Autodesk Fusion 360 part; units mm, degrees
sketch "Skizze1" plane through (0, 0, 0) normal (0, 0, 1) x (1, 0, 0)
  line L0 (0, 0) -> (57, 0)
  line L1 (57, 0) -> (57, 87)
  line L2 (57, 87) -> (0, 87)
  line L3 (0, 87) -> (0, 0)
  dimension "d1" = 57
  dimension "d2" = 87
extrude "Extrusion1" add sketch "Skizze1" along normal blind 1.75
fillet "Abrundung1" radius 2 4 edges at (0, 0, 0.875) (57, 0, 0.875) (57, 87, 0.875) (0, 87, 0.875)
sketch "Skizze2" plane through (0, 0, 1.75) normal (0, 0, 1) x (-1, 0, 0)
  arc A0 (-2, -87) -> (0, -85) centre (-2, -85) ccw
  line L0 (0, -85) -> (0, -2)
  arc A1 (0, -2) -> (-2, 0) centre (-2, -2) ccw
  line L1 (-2, 0) -> (-55, 0)
  arc A2 (-55, 0) -> (-57, -2) centre (-55, -2) ccw
  line L2 (-57, -2) -> (-57, -85)
  arc A3 (-57, -85) -> (-55, -87) centre (-55, -85) ccw
  line L3 (-55, -87) -> (-2, -87)
  line L4 (-5.5896, -49.2464) -> (-5.5896, -40.6115)
  line L5 (-5.5896, -40.6115) -> (-12.2493, -39.4747)
  spline S0 degree 3 poles (-12.2493, -39.4747) (-12.5241, -38.6458) (-12.8509, -37.8501) (-13.2393, -37.0827) knots 0 0 0 0 1 1 1 1
  line L6 (-13.2393, -37.0827) -> (-9.3316, -31.5693)
  line L7 (-9.3316, -31.5693) -> (-15.4418, -25.459)
  line L8 (-15.4418, -25.459) -> (-20.9932, -29.3904)
  spline S1 degree 3 poles (-20.9932, -29.3904) (-21.7416, -29.0162) (-22.5231, -28.7083) (-23.3331, -28.4478) knots 0 0 0 0 1 1 1 1
  line L9 (-23.3331, -28.4478) -> (-24.4794, -21.7171)
  line L10 (-24.4794, -21.7171) -> (-33.1143, -21.7171)
  line L11 (-33.1143, -21.7171) -> (-34.2747, -28.5189)
  spline S2 degree 3 poles (-34.2747, -28.5189) (-35.0515, -28.7794) (-35.7952, -29.092) (-36.5152, -29.4567) knots 0 0 0 0 1 1 1 1
  line L12 (-36.5152, -29.4567) -> (-42.1565, -25.459)
  line L13 (-42.1565, -25.459) -> (-48.2668, -31.5693)
  line L14 (-48.2668, -31.5693) -> (-44.2454, -37.2438)
  spline S3 degree 3 poles (-44.2454, -37.2438) (-44.5959, -37.9495) (-44.8801, -38.679) (-45.1359, -39.4321) knots 0 0 0 0 1 1 1 1
  line L15 (-45.1359, -39.4321) -> (-52.0087, -40.6068)
  line L16 (-52.0087, -40.6068) -> (-52.0087, -49.2464)
  line L17 (-52.0087, -49.2464) -> (-45.1311, -50.4211)
  spline S4 degree 3 poles (-45.1311, -50.4211) (-44.8801, -51.179) (-44.5911, -51.8989) (-44.2406, -52.6047) knots 0 0 0 0 1 1 1 1
  line L18 (-44.2406, -52.6047) -> (-48.262, -58.2839)
  line L19 (-48.262, -58.2839) -> (-42.1565, -64.3895)
  line L20 (-42.1565, -64.3895) -> (-36.5152, -60.3965)
  spline S5 degree 3 poles (-36.5152, -60.3965) (-35.7952, -60.7612) (-35.0515, -61.0691) (-34.2795, -61.3343) knots 0 0 0 0 1 1 1 1
  line L21 (-34.2795, -61.3343) -> (-33.1143, -68.1362)
  line L22 (-33.1143, -68.1362) -> (-24.4746, -68.1362)
  line L23 (-24.4746, -68.1362) -> (-23.3236, -61.4054)
  spline S6 degree 3 poles (-23.3236, -61.4054) (-22.5137, -61.1401) (-21.7368, -60.837) (-20.9885, -60.4628) knots 0 0 0 0 1 1 1 1
  line L24 (-20.9885, -60.4628) -> (-15.4418, -64.3942)
  line L25 (-15.4418, -64.3942) -> (-9.3316, -58.2887)
  line L26 (-9.3316, -58.2887) -> (-13.2346, -52.7752)
  spline S7 degree 3 poles (-13.2346, -52.7752) (-12.8414, -52.0079) (-12.5193, -51.2121) (-12.2446, -50.3832) knots 0 0 0 0 1 1 1 1
  line L27 (-12.2446, -50.3832) -> (-5.5896, -49.2464)
  spline S8 degree 3 poles (-28.695, -53.2157) (-33.2706, -53.2157) (-36.9841, -49.5069) (-36.9841, -44.9266) knots 0 0 0 0 1 1 1 1
  spline S9 degree 3 poles (-36.9841, -44.9266) (-36.9841, -40.351) (-33.2706, -36.6375) (-28.695, -36.6375) knots 0 0 0 0 1 1 1 1
  spline S10 degree 3 poles (-28.695, -36.6375) (-24.1146, -36.6375) (-20.4058, -40.351) (-20.4058, -44.9266) knots 0 0 0 0 1 1 1 1
  spline S11 degree 3 poles (-20.4058, -44.9266) (-20.4058, -49.5069) (-24.1194, -53.2157) (-28.695, -53.2157) knots 0 0 0 0 1 1 1 1
extrude "Extrusion2" cut sketch "Skizze2" against normal blind 0.4 contours L4 L5 S0 L6 L7 L8 S1 L9 L10 L11 S2 L12 L13 L14 S3 L15 L16 L17 S4 L18 L19 L20 S5 L21 L22 L23 S6 L24 L25 L26 S7 L27
extrude "Extrusion3" cut 1 faces at (19, 57.3333, 0) along direction (0, 0, 1) blind 0.2
extrude "Extrusion4" cut 1 faces at (19, 57.3333, 0.2) along direction (0, 0, 1) blind 0.05
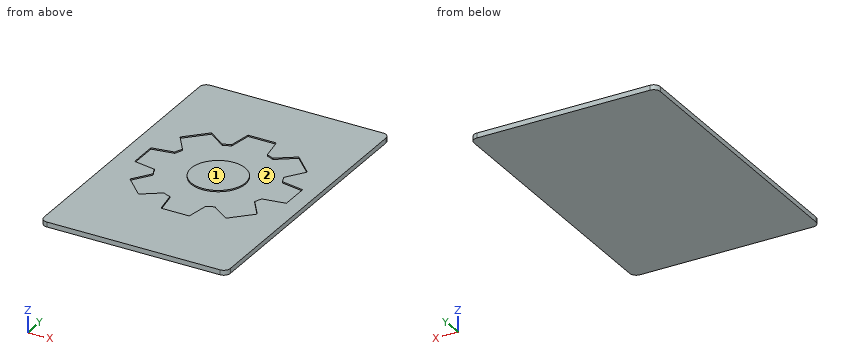
Geometry check sheet. Reference: the model listing, model coordinates, mm. Face numbers are marked on the shaded views. Give positions to 0.01 mm unless a question says otherwise; leave off trailing zeros. Write each loop counter-clockwise with the first axis right and the second up, starting at its lowest first coordinate (ties: lowest second). Pieces come first, ordered by that corner, then holes.
1) Cross-section at A-A (x = 51). Record the boundary of the cut face in (y, z), plus the area to 3 significant figures.
Values follow:
outline: (0, 0.25) - (87, 0.25) - (87, 1.75) - (49.42, 1.75) - (49.42, 1.35) - (40.43, 1.35) - (40.43, 1.75) - (0, 1.75) - close
area: 127 mm2
2) Go/stop test with a flat-tipped pin: pin 1 Ø1 at (x, y) = (27.5, 55) entering from +Z. Record where the tip stops, or that it passes through.
Values follow:
pin 1: stops at z = 1.35
3) Cross-section at B-B (x = 11). Record the boundary of the cut face in (y, z).
Values follow:
outline: (0, 0.25) - (87, 0.25) - (87, 1.75) - (59.96, 1.75) - (59.96, 1.35) - (55.93, 1.35) - (55.93, 1.75) - (50.17, 1.75) - (50.17, 1.35) - (39.69, 1.35) - (39.69, 1.75) - (33.92, 1.75) - (33.92, 1.35) - (29.9, 1.35) - (29.9, 1.75) - (0, 1.75) - close
4) Release check for a two-part mould opening along X. For the marked faces 1 and 2 record: released by +X, released by -X, zero draft, split by the parting line, or undercut.
Values follow:
face 1: zero draft
face 2: undercut
5) Thickness scan on line 1 (Z direction, x = 13, y = 42.5); line 2 (Y direction, x = 18.5, z = 1.55); line 3 (Y direction, x = 20, z = 1.65). Record the ranges inside material, lowest first.
Values follow:
line 1: z = 0.25 to 1.35
line 2: y = 0 to 27.62, 62.23 to 87
line 3: y = 0 to 28.69, 61.16 to 87
